Here's the drawing with two shaded views (mm, measured from the low corner). I have some questions. Coordinates: 2 decimals unless noted, no trailing zeros. Write each loop counter-clockwise with the first axis right and the second up, starting at its lowest first coordinate (ties: lowest second). Pieces come first, ordered by that corner, then holes. Notation, with made-up numbers: (34.5, 78.5) -> (67.5, 78.5) arc R28 cw to (67.5, 115.5) -> close; hole circle Ø7 at (26, 45). An arc over 180 degrees is marked (long way). Use one line per item in the form item = value.
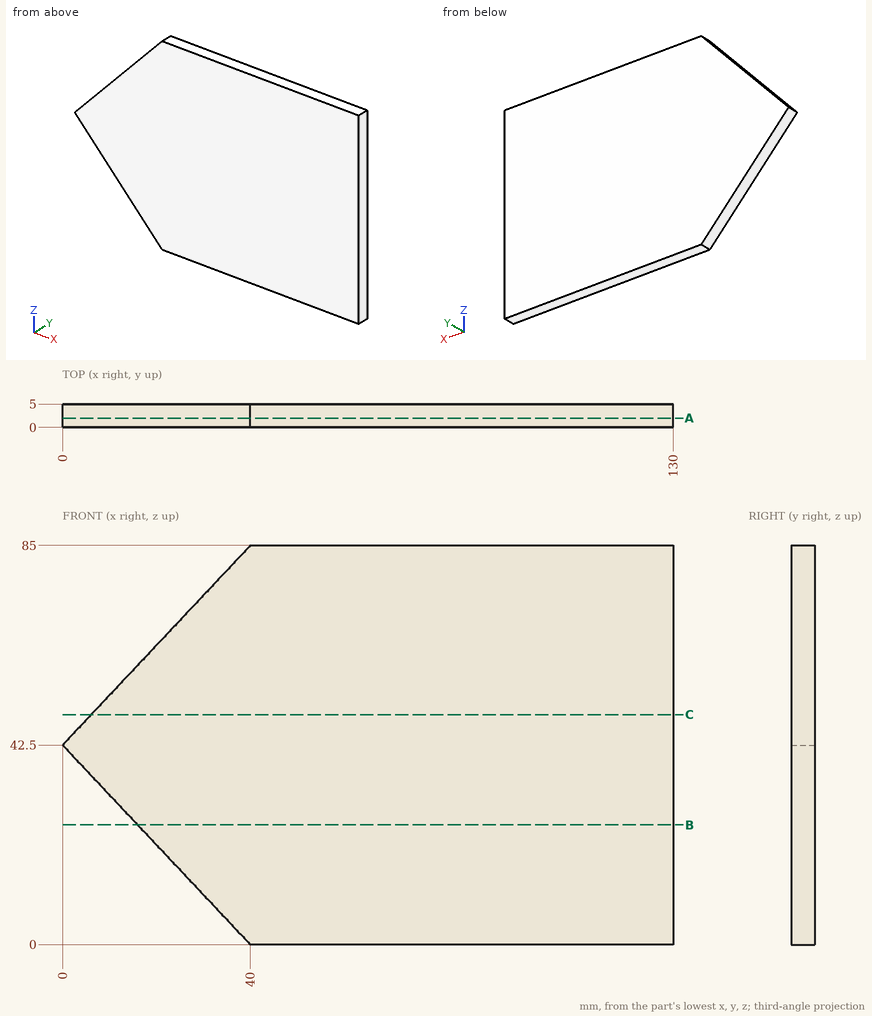
Q1. Suppose I cut it at B-B (z = 25.5). Write out the boundary of the cut face in (x, y), then the cut area to 3 significant figures.
Return value:
outline = (16, 0) -> (130, 0) -> (130, 5) -> (16, 5) -> close
area = 570 mm2
Q2. Will this pin go through, and if not, where does the flat tip stop? pin 1 (1 mm diameter, centred on y = 3.5, z = 70.5, fed in from -X).
Return value:
pin_1 = 25.88
Q3. Suppose I cut it at A-A (y = 2). Write out the boundary of the cut face in (x, z), then the cut area to 3 significant figures.
Return value:
outline = (0, 42.5) -> (40, 0) -> (130, 0) -> (130, 85) -> (40, 85) -> close
area = 9,350 mm2
Q4. Suppose I cut it at C-C (z = 49). Write out the boundary of the cut face in (x, y), then the cut area to 3 significant figures.
Return value:
outline = (6.12, 0) -> (130, 0) -> (130, 5) -> (6.12, 5) -> close
area = 619 mm2
Q5. If I drill on line 1 (X direction, y = 4.3, z = 77); line 2 (Z direction, x = 5, y = 1); line 3 (Z direction, x = 13.5, y = 3.95), over which ranges is the centre line in solid material (lowest first)? Write a range as from..to.
Return value:
line_1 = 32.47..130
line_2 = 37.19..47.81
line_3 = 28.16..56.84
